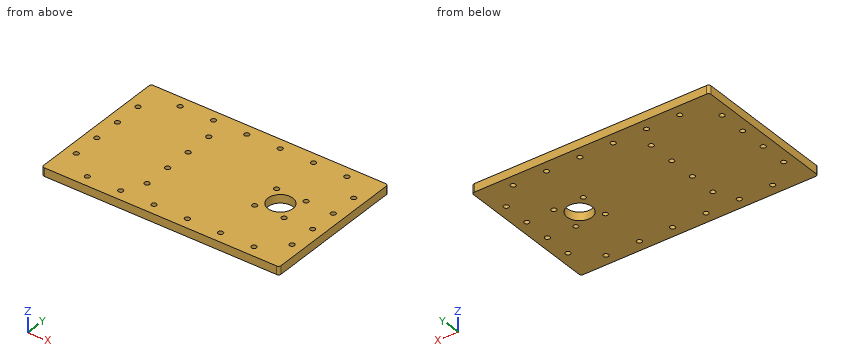
from build123d import *

# Parameters (mm, degrees)
SKETCH_W   = 285
SKETCH_H   = 175
SKETCH_R   = 15
SKETCH_R_2 = 3
PAD_DEPTH  = 10
FILLET_R   = 3


with BuildPart() as part:
    # Sketch → Pad (new body)
    with BuildSketch(Plane.XY):
        with Locations((57.5, 100)):
            Rectangle(SKETCH_W, SKETCH_H)
        with Locations((136, 100)):
            Circle(SKETCH_R, mode=Mode.SUBTRACT)
        with Locations((118.32233, 117.67767)):
            Circle(SKETCH_R_2, mode=Mode.SUBTRACT)
        with Locations((153.67767, 117.67767)):
            Circle(SKETCH_R_2, mode=Mode.SUBTRACT)
        with Locations((118.32233, 82.32233)):
            Circle(SKETCH_R_2, mode=Mode.SUBTRACT)
        with Locations((153.67767, 82.32233)):
            Circle(SKETCH_R_2, mode=Mode.SUBTRACT)
        with Locations((40, 25.5)):
            Circle(SKETCH_R_2, mode=Mode.SUBTRACT)
        with Locations((160, 25.5)):
            Circle(SKETCH_R_2, mode=Mode.SUBTRACT)
        with Locations((80, 25.5)):
            Circle(SKETCH_R_2, mode=Mode.SUBTRACT)
        with Locations((120, 25.5)):
            Circle(SKETCH_R_2, mode=Mode.SUBTRACT)
        with Locations((40, 174.5)):
            Circle(SKETCH_R_2, mode=Mode.SUBTRACT)
        with Locations((80, 174.5)):
            Circle(SKETCH_R_2, mode=Mode.SUBTRACT)
        with Locations((120, 174.5)):
            Circle(SKETCH_R_2, mode=Mode.SUBTRACT)
        with Locations((160, 174.5)):
            Circle(SKETCH_R_2, mode=Mode.SUBTRACT)
        with Locations((13, 149.5)):
            Circle(SKETCH_R_2, mode=Mode.SUBTRACT)
        with Locations((13, 116.5)):
            Circle(SKETCH_R_2, mode=Mode.SUBTRACT)
        with Locations((13, 83.5)):
            Circle(SKETCH_R_2, mode=Mode.SUBTRACT)
        with Locations((13, 50.5)):
            Circle(SKETCH_R_2, mode=Mode.SUBTRACT)
        with Locations((187, 149.5)):
            Circle(SKETCH_R_2, mode=Mode.SUBTRACT)
        with Locations((187, 116.5)):
            Circle(SKETCH_R_2, mode=Mode.SUBTRACT)
        with Locations((187, 83.5)):
            Circle(SKETCH_R_2, mode=Mode.SUBTRACT)
        with Locations((187, 50.5)):
            Circle(SKETCH_R_2, mode=Mode.SUBTRACT)
        with Locations((-72, 149.5)):
            Circle(SKETCH_R_2, mode=Mode.SUBTRACT)
        with Locations((-72, 116.5)):
            Circle(SKETCH_R_2, mode=Mode.SUBTRACT)
        with Locations((-72, 83.5)):
            Circle(SKETCH_R_2, mode=Mode.SUBTRACT)
        with Locations((-72, 50.5)):
            Circle(SKETCH_R_2, mode=Mode.SUBTRACT)
        with Locations((-40, 25.5)):
            Circle(SKETCH_R_2, mode=Mode.SUBTRACT)
        with Locations((0, 25.5)):
            Circle(SKETCH_R_2, mode=Mode.SUBTRACT)
        with Locations((-40, 174.5)):
            Circle(SKETCH_R_2, mode=Mode.SUBTRACT)
        with Locations((0, 174.5)):
            Circle(SKETCH_R_2, mode=Mode.SUBTRACT)
    extrude(amount=PAD_DEPTH)

    # Fillet
    fillet_edges = [part.edges().sort_by_distance(p)[0] for p in [
        (200, 12.5, 5),
        (200, 187.5, 5),
        (-85, 12.5, 5),
        (-85, 187.5, 5),
    ]]
    fillet(fillet_edges, radius=FILLET_R)


solid = part.part
Source: CAD feature listing. Evaluate the final solid. Frame: model axes, mm. Coordinates: 2 decimals unless noted, no trailing zeros. Order: outer loops, then holes, each group sorted by start corner. A loop starts at its lowest first (then second) coordinate and runs counter-clockwise, first axis right, second up. Notation, with made-up numbers: M 25.25,22 L 50.25,22 A33 cw 50.25,55 Z; hole C 49.5,-26 d11. An arc over 180 degrees is marked long. Write each question's results on one line, items separated by ' | '. Start each with the question number.
1. Material intervals for L1, parallel to Y at x = 40, z = 5.75; L2, parallel to Y at x = 187, z = 6.25; L3, parallel to X at y = 117, z = 8.5, sorted ascending.
2. Section C-C, the plane y = 174.5. Return the cut outline in (x, z), then the cut area to 3 significant figures.
3. Section D-D, the plane x = 187. Return the cut outline in (y, z), then the cut area to 3 significant figures.
4. Section A-A, the plane y = 50.5. Return the cut outline in (x, z).
5. Section B-B, the plane x = 80. Return the cut outline in (y, z).
6. Pin query (flat end, axial travel): pin 1 (3.5 mm diameter, centred on x = 0, y = 174.5, fed in from -Z). Return the tip coordinate at first contact, or that it passes through.
Solution:
1) L1: 12.5 to 22.5, 28.5 to 171.5, 177.5 to 187.5 | L2: 12.5 to 47.5, 53.5 to 80.5, 86.5 to 113.5, 119.5 to 146.5, 152.5 to 187.5 | L3: -85 to -74.96, -69.04 to 10.04, 15.96 to 115.4, 121.24 to 150.76, 156.6 to 184.04, 189.96 to 200
2) outline: M -85,0 L -43,0 L -43,10 L -85,10 Z; M -37,0 L -3,0 L -3,10 L -37,10 Z; M 3,0 L 37,0 L 37,10 L 3,10 Z; M 43,0 L 77,0 L 77,10 L 43,10 Z; M 83,0 L 117,0 L 117,10 L 83,10 Z; M 123,0 L 157,0 L 157,10 L 123,10 Z; M 163,0 L 200,0 L 200,10 L 163,10 Z | area: 2,490 mm²
3) outline: M 12.5,0 L 47.5,0 L 47.5,10 L 12.5,10 Z; M 53.5,0 L 80.5,0 L 80.5,10 L 53.5,10 Z; M 86.5,0 L 113.5,0 L 113.5,10 L 86.5,10 Z; M 119.5,0 L 146.5,0 L 146.5,10 L 119.5,10 Z; M 152.5,0 L 187.5,0 L 187.5,10 L 152.5,10 Z | area: 1,510 mm²
4) outline: M -85,0 L -75,0 L -75,10 L -85,10 Z; M -69,0 L 10,0 L 10,10 L -69,10 Z; M 16,0 L 184,0 L 184,10 L 16,10 Z; M 190,0 L 200,0 L 200,10 L 190,10 Z
5) outline: M 12.5,0 L 22.5,0 L 22.5,10 L 12.5,10 Z; M 28.5,0 L 171.5,0 L 171.5,10 L 28.5,10 Z; M 177.5,0 L 187.5,0 L 187.5,10 L 177.5,10 Z
6) pin 1: through
